```python
from build123d import *

# Parameters (mm, degrees)
F1_DEPTH = 25
F3_DEPTH = 80
F5_DEPTH = 80


with BuildPart() as f1:
    # F0 (on Front) → F1 (new body)
    with BuildSketch(Plane.XZ):
        Polygon((-80, 0), (0, 0), (0, 33.64), (0, 80), (-80, 80), align=None)
    extrude(amount=F1_DEPTH)

    # F2 (on face) → F3 (cut)
    with BuildSketch(Plane(origin=(0, 0, 0), x_dir=(1, 0, 0), z_dir=(0, 0, -1))):
        Polygon((-33.64, 25), (-46.36, 25), (-50, 15), (-30, 15), align=None)
    extrude(amount=-F3_DEPTH, mode=Mode.SUBTRACT)

    # F4 (on Right) → F5 (cut)
    with BuildSketch(Plane.YZ):
        Polygon((-25.113055, 33.64), (-15, 30), (-15, 50), (-25.113055, 46.36), align=None)
    extrude(amount=-F5_DEPTH, mode=Mode.SUBTRACT)


solid = f1.part
```
The listing builds one solid part. Answer for the finished solid, in the listing's coordinates (mm). A direction names the side the tool comes from. Coordinates: 2 decimals unless noted, no trailing zeros. Loops run counter-clockwise (first coordinate to the right, second up) from the corner with the lowest first, then second, coordinate; pieces in that order, holes last. Notation, with made-up numbers: (60, 50.25) - (83, 50.25) arc R20 cw to (83, 87.25) - close; hole circle Ø8 at (78, -11.75). An arc over 180 degrees is marked (long way). Write item = value, one per line.
1) Section C-C (x = -25.5) is taken. Determine the outline of the cut face in (y, z).
Responses:
outline = (-25, 0) - (0, 0) - (0, 80) - (-25, 80) - (-25, 46.4) - (-15, 50) - (-15, 30) - (-25, 33.6) - close
2) Section D-D (x = -37.5) is taken. Determine the outline of the cut face in (y, z), plus the area to 3 significant figures.
Responses:
outline = (-15, 0) - (0, 0) - (0, 80) - (-15, 80) - close
area = 1,200 mm^2
3) Determine the mould class of faces 5 (the face through (-17, -25, 17)), 6 (the face through (-31.795, -19.93, 62.965)), 7 (the face through (-39, -12, 80)) for opening direction Y: pulls with the +Y half, pulls with the -Y half, needs draft (parallel to the pull), parting line crosses it, or undercut.
Responses:
face_5 = pulls with the -Y half
face_6 = undercut
face_7 = needs draft
4) Which of the six approach directions +Z, -Z, +X, -X, +Y, -Y give full straight-line access (tool end or side, diameter ignored) to faces 1 (the face through (-31.795, -19.93, 16.564)), 2 (the face through (-41, -12, 0)), 3 (the face through (-16.585, -20.07, 31.825)), 4 (the face through (-41, -15, 39))?
Responses:
face_1 = +Z, -Z
face_2 = -Z, +X, -X, +Y, -Y
face_3 = +X, -X
face_4 = none
5) Find the intervals of material crossed by line 1 along X through (y, z) = (-17.25, 65); line 2 along X through (y, z) = (-18.5, 15.5); line 3 along Z through (x, y) = (-16, -18), in increasing order.
Responses:
line_1 = -80 to -49.18, -30.82 to 0
line_2 = -80 to -48.73, -31.27 to 0
line_3 = 0 to 31.08, 48.92 to 80
6) Section B-B (y = -16.25) is taken. Determine the outline of the cut face in (x, z) (3 decimals).
Responses:
outline = (-80, 0) - (-49.545, 0) - (-49.545, 30.45) - (-80, 30.45) - close; (-80, 49.55) - (-49.545, 49.55) - (-49.545, 80) - (-80, 80) - close; (-30.455, 0) - (0, 0) - (0, 30.45) - (-30.455, 30.45) - close; (-30.455, 49.55) - (0, 49.55) - (0, 80) - (-30.455, 80) - close
7) This flat-tipped pin is pushed along its axis until it touches: P1, Ø2, axis at y = -18, z = 69.5, coming from the +X side. Where does it stop, or does it pass through?
Responses:
P1 = 0
8) Section A-A (z = 24.5) is taken. Determine the outline of the cut face in (x, y).
Responses:
outline = (-80, -25) - (-46.36, -25) - (-50, -15) - (-30, -15) - (-33.64, -25) - (0, -25) - (0, 0) - (-80, 0) - close
